```python
from build123d import *

# Parameters (mm, degrees)
SKETCH_1_W          = 64
SKETCH_1_H          = 36.2
SKETCH_1_R          = 1.5
SKETCH_1_W_2        = 42
SKETCH_1_H_2        = 22
EXTRUDE_1_DEPTH     = 3
SKETCH_2_W          = 18
SKETCH_2_H          = 22
EXTRUDE_2_DEPTH     = 3
SKETCH_3_R          = 1.5
CUT_EXTRUDE_1_DEPTH = 3
FILLET_1_R          = 10
FILLET_2_R          = 3


with BuildPart() as part:
    # 草图1 → 凸台-拉伸1 (new body)
    with BuildSketch(Plane(origin=(0, 0, 0), x_dir=(1, 0, 0), z_dir=(0, 1, 0))):
        Rectangle(SKETCH_1_W, SKETCH_1_H)
        with Locations(Location((22.14, 9.1, 0), (0, 0, 270))):
            Circle(SKETCH_1_R, mode=Mode.SUBTRACT)
        with Locations(Location((22.14, -0.9, 0), (0, 0, 90))):
            Circle(SKETCH_1_R, mode=Mode.SUBTRACT)
        with Locations(Location((-27.36, -0.9, 0), (0, 0, 270))):
            Circle(SKETCH_1_R, mode=Mode.SUBTRACT)
        with Locations(Location((-27.36, 9.1, 0), (0, 0, 90))):
            Circle(SKETCH_1_R, mode=Mode.SUBTRACT)
        with Locations(Location((9, -13.6, 0), (0, 0, 270))):
            Circle(SKETCH_1_R, mode=Mode.SUBTRACT)
        with Locations(Location((-9, -13.6, 0), (0, 0, 90))):
            Circle(SKETCH_1_R, mode=Mode.SUBTRACT)
        with Locations((-2.61, 4.1)):
            Rectangle(SKETCH_1_W_2, SKETCH_1_H_2, mode=Mode.SUBTRACT)
    extrude(amount=EXTRUDE_1_DEPTH)

    # 草图2 → 凸台-拉伸2 (add)
    with BuildSketch(Plane(origin=(0, 3, 0), x_dir=(1, 0, 0), z_dir=(0, 1, 0))):
        with Locations((9.39, 4.1)):
            Rectangle(SKETCH_2_W, SKETCH_2_H)
    extrude(amount=-EXTRUDE_2_DEPTH)

    # 草图3 → 切除-拉伸1 (cut)
    with BuildSketch(Plane(origin=(0, 3, 0), x_dir=(1, 0, 0), z_dir=(0, 1, 0))):
        with Locations(Location((12.39, 4.1, 0), (0, 0, 270))):
            Circle(SKETCH_3_R)
    extrude(amount=-CUT_EXTRUDE_1_DEPTH, mode=Mode.SUBTRACT)

    # 圆角1
    fillet_1_edges = [part.edges().sort_by_distance(p)[0] for p in [
        (32, 1.5, 18.1),
        (-32, 1.5, 18.1),
        (-32, 1.5, -18.1),
        (32, 1.5, -18.1),
    ]]
    fillet(fillet_1_edges, radius=FILLET_1_R)

    # 圆角2
    fillet_2_edges = [part.edges().sort_by_distance(p)[0] for p in [
        (-23.61, 1.5, -15.1),
        (-23.61, 1.5, 6.9),
        (0.39, 1.5, -15.1),
        (0.39, 1.5, 6.9),
    ]]
    fillet(fillet_2_edges, radius=FILLET_2_R)


solid = part.part
```
Can you work these out from the model? Positions are in its coordinate system, mm. A direction names the side the tool comes from. Coordinates: 2 decimals unless noted, no trailing zeros. Loops run counter-clockwise (first coordinate to the right, second up) from the corner with the lowest first, then second, coordinate; pieces in that order, holes last. Notation, with made-up numbers: (-21, 73) - (17, 73) arc R37 ccw to (17, 109) - close; hole circle Ø11 at (4, 20). An arc over 180 degrees is marked (long way). Answer as CSV lines item,"result". Start each with the question number.
1) I need wall thicknesses on line 1 (X direction, y = 2.05, z = -3); line 2 (X direction, y = 0.55, z = 2); line 3 (X direction, y = 2, z = -4.1). Which ranges of each line are inside material? Lowest first, please. Write a range as from..to.
2) For pin 1 (1 mm diameter, centred on y = 2, z = -10.5, fed in from -X), with a flat end and sliding along its axis, tell me the tip position at first contact or that it passes through.
3) Thinking about a two-plate mould opening in X: for faces 3 (the flat face through (32, 1, 0)), 4 (the flat face through (7, 0, 0)), 5 (the cylindrical face through (-29.15, 1.52, -15.09)), 6 (the cylindrical face through (-22.71, 1.52, -14.24)), which applies, pulls with the +X half, pulls with the -X half, needs draft (parallel to the pull), parting line crosses it, or undercut?
4) Suppose I cut it at D-D (y = 1.8). Count the separate pieces of the cut face and the enclosed holes in it, plus the area to 3 significant figures.
5) Suppose I cut it at A-A (x = -18). Please give me the cut outline in (y, z), plus the area to 3 significant figures.
6) Which directions (+Z, -Z, +X, -X, +Y, -Y) give clear straight access to the entire face, cutting with the end or side of a thin tool? Please do faces 1 (the cylindrical face through (-0.47, 1.48, 6)), 2 (the flat face through (0, 1, -18.1)).
7) Suppose I cut it at C-C (x = -9). Please give me the cut outline in (y, z), plus the area to 3 significant figures.
8) Suppose I cut it at B-B (z = 0.9). Please give me the cut outline in (x, y), plus the area to 3 significant figures.
Check result:
1,line 1,"x = -32..-23.61, 0.39..11.37, 13.41..32"
1,line 2,"x = -32..-28.38, -26.34..-23.61, 0.39..21.12, 23.16..32"
1,line 3,"x = -32..-23.61, 0.39..10.89, 13.89..32"
2,pin 1,"stops at x = -31.82"
3,face 3,"pulls with the +X half"
3,face 4,"needs draft"
3,face 5,"pulls with the -X half"
3,face 6,"undercut"
4,separate pieces,"1"
4,enclosed holes,"8"
4,area,"1,660 mm²"
5,outline,"(0, -18.1) - (3, -18.1) - (3, -15.1) - (0, -15.1) - close; (0, 6.9) - (3, 6.9) - (3, 18.1) - (0, 18.1) - close"
5,area,"42.6 mm²"
6,face 1,"+Y, -Y"
6,face 2,"-Z, +X, -X, +Y, -Y"
7,outline,"(0, -18.1) - (3, -18.1) - (3, -15.1) - (0, -15.1) - close; (0, 6.9) - (3, 6.9) - (3, 12.1) - (0, 12.1) - close; (0, 15.1) - (3, 15.1) - (3, 18.1) - (0, 18.1) - close"
7,area,"33.6 mm²"
8,outline,"(-32, 0) - (-28.86, 0) - (-28.86, 3) - (-32, 3) - close; (-25.86, 0) - (-23.61, 0) - (-23.61, 3) - (-25.86, 3) - close; (0.39, 0) - (20.64, 0) - (20.64, 3) - (0.39, 3) - close; (23.64, 0) - (32, 0) - (32, 3) - (23.64, 3) - close"
8,area,"102 mm²"
